```python
from build123d import *

# Parameters (mm, degrees)
SKETCH1_R           = 9.525
BOSS_EXTRUDE1_DEPTH = 139.7
FILLET1_R           = 9.525


with BuildPart() as part:
    # Sketch1 → Boss-Extrude1 (new body)
    with BuildSketch(Plane.XY):
        Circle(SKETCH1_R)
    extrude(amount=BOSS_EXTRUDE1_DEPTH)

    # Fillet1
    fillet1_edges = [part.edges().sort_by_distance(p)[0] for p in [
        (-9.525, 0, 0),
    ]]
    fillet(fillet1_edges, radius=FILLET1_R)

    # Sketch2 → 3/8-16 Tapped Hole1 (revolve, cut)
    with BuildSketch(Plane(origin=(0, 0, 139.7), x_dir=(0, -1, 0), z_dir=(1, 0, 0))):
        Polygon((0, 0), (0, 42.084865582), (3.96875, 39.7002), (3.96875, 31.75), (4.7625, 31.75), (4.7625, 0.635), (5.3975, 0), align=None)
    revolve(axis=Axis((0, 0, 146.05), (0, 0, -1)), mode=Mode.SUBTRACT)


solid = part.part
```
Work out the finished part from the listing and answer in its coordinate system (mm). Coordinates: 2 decimals unless noted, no trailing zeros. Write each loop counter-clockwise with the first axis right and the second up, starting at its lowest first coordinate (ties: lowest second). Pieces come first, ordered by that corner, then holes.
Q1. Determine the mould class of faces 1 (the face through (4, -4, 139.7)), 2 (the face through (2.9, 3.78, 123.73)), 3 (the face through (-7.559, -5.796, 73.701)) for opening direction X: released by +X, released by -X, zero draft, split by the parting line, or undercut.
Q2. A cutting plane is placed at A-A, the plane z = 23.5. Give the vertices of the cut face in (x, y) (3 decimals).
Q3. A cutting plane is placed at B-B, the plane y = 6.75. Give the vertices of the cut face in (x, z) (3 decimals).
Q4. Find the intervals of material crossed by line 1 (Y direction, x = 0, z = 132.5) (1 decimal); line 2 (Y direction, x = 0, z = 102.5) (3 decimals); line 3 (X direction, y = -8.25, z = 111), in increasing order.
Q5. Each of these flat-tipped pins is pushed along its axis until it touches: pin 1 Ø3 at (x, z) = (2.5, 67.5) entering from +Y; pin 2 Ø1 at (y, z) = (2, 45) entering from +X; pin 3 Ø3 at (x, y) = (1.5, 2.5) entering from +Z. Where does it stop, or does it pass through?
Findings below:
1. face 1: zero draft
1. face 2: undercut
1. face 3: split by the parting line
2. outline: circle Ø19.05 at (0, 0)
3. outline: (-6.72, 9.525) arc R6.72 ccw to (6.72, 9.525) - (6.72, 139.7) - (-6.72, 139.7) - close
4. line 1: y = -9.5 to -4.8, 4.8 to 9.5
4. line 2: y = -9.525 to -3.969, 3.969 to 9.525
4. line 3: x = -4.76 to 4.76
5. pin 1: stops at y = 9.47
5. pin 2: stops at x = 9.41
5. pin 3: stops at z = 107.95
